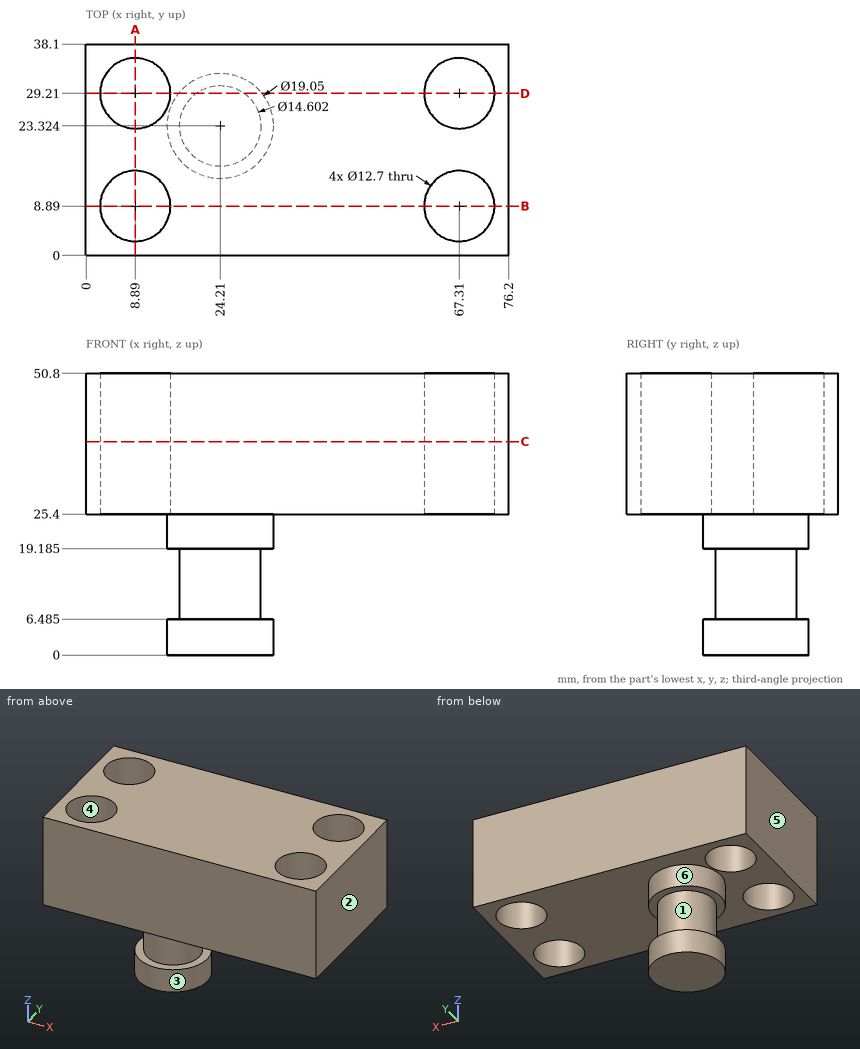
Answer from the drawing. Dimensions are ordinates in mm from the lowest x, y and z of the part. A direction names the side the tool comes from. Round coordinates to 2 decimals unless told otherwise and drop trailing zeros. Write each loop counter-clockwise with the first axis right and the second up, starting at its lowest first coordinate (ties: lowest second). Pieces come first, ordered by that corner, then holes. Notation, with made-up numbers: (13, -32) - (18, -32) arc R24 ccw to (18, -6) - close; hole circle Ø8 at (84.5, -1). An arc over 180 degrees is marked (long way). Use a Markdown table: item, result.
(1) The mould has two halves that part along Y. Classify the marked faces 4, 5 and 6: released by +Y, released by -Y, zero draft, split by the parting line, or undercut.
Reported:
| item | result |
|---|---|
| face 4 | undercut |
| face 5 | zero draft |
| face 6 | split by the parting line |
(2) The part is cut by section D-D (y = 29.21). Write down the section's boundary in (x, z) (1 decimal), then the cut area to 3 significant figures.
Reported:
| item | result |
|---|---|
| outline | (0, 25.4) - (2.5, 25.4) - (2.5, 50.8) - (0, 50.8) - close; (15.2, 25.4) - (16.7, 25.4) - (16.7, 19.2) - (19.9, 19.2) - (19.9, 6.5) - (16.7, 6.5) - (16.7, 0) - (31.7, 0) - (31.7, 6.5) - (28.5, 6.5) - (28.5, 19.2) - (31.7, 19.2) - (31.7, 25.4) - (61, 25.4) - (61, 50.8) - (15.2, 50.8) - close; (73.7, 25.4) - (76.2, 25.4) - (76.2, 50.8) - (73.7, 50.8) - close |
| area | 1,590 mm2 |
(3) The part is cut by section A-A (x = 8.89). Write down the section's boundary in (y, z).
Reported:
| item | result |
|---|---|
| outline | (0, 25.4) - (2.54, 25.4) - (2.54, 50.8) - (0, 50.8) - close; (15.24, 25.4) - (22.86, 25.4) - (22.86, 50.8) - (15.24, 50.8) - close; (35.56, 25.4) - (38.1, 25.4) - (38.1, 50.8) - (35.56, 50.8) - close |
(4) Straight lines are drawn through the part: line 1 along Y through (x, z) = (67.31, 39.25); line 2 along X through (y, z) = (29, 35); line 3 along X through (y, z) = (31, 42.5). For each, find the intervals that lie inside material, in ascending order. Write a range as [from, to].
Reported:
| item | result |
|---|---|
| line 1 | [0, 2.54], [15.24, 22.86], [35.56, 38.1] |
| line 2 | [0, 2.54], [15.24, 60.96], [73.66, 76.2] |
| line 3 | [0, 2.8], [14.98, 61.22], [73.4, 76.2] |
(5) Which of the six approach directions +Z, -Z, +X, -X, +Y, -Y give full straight-line access (tool end or side, diameter ignored) to the marked faces 1, 2 and 3?
Reported:
| item | result |
|---|---|
| face 1 | none |
| face 2 | +Z, -Z, +X, +Y, -Y |
| face 3 | -Z |
(6) Each of these flat-tipped pins is pushed along its axis until it touches: pin 1 Ø5 at (x, z) = (27, 6) entering from +Y (1 decimal); pin 2 Ø20.5 at (x, y) = (67.31, 29.21) entering from -Z. Where does it stop, or does it pass through?
Reported:
| item | result |
|---|---|
| pin 1 | y = 32.8 |
| pin 2 | z = 25.4 |
(7) The part is cut by section C-C (z = 38.5). Write down the section's boundary in (x, y), then the cut area to 3 significant figures.
Reported:
| item | result |
|---|---|
| outline | (0, 0) - (76.2, 0) - (76.2, 38.1) - (0, 38.1) - close; hole circle Ø12.7 at (8.89, 8.89); hole circle Ø12.7 at (8.89, 29.21); hole circle Ø12.7 at (67.31, 8.89); hole circle Ø12.7 at (67.31, 29.21) |
| area | 2,400 mm2 |
(8) The part is cut by section B-B (y = 8.89). Write down the section's boundary in (x, z).
Reported:
| item | result |
|---|---|
| outline | (0, 25.4) - (2.54, 25.4) - (2.54, 50.8) - (0, 50.8) - close; (15.24, 25.4) - (60.96, 25.4) - (60.96, 50.8) - (15.24, 50.8) - close; (73.66, 25.4) - (76.2, 25.4) - (76.2, 50.8) - (73.66, 50.8) - close |
